Autodesk Inventor part; units mm, degrees
ref_plane "YZ Plane" through (0, 0, 0) normal (1, 0, 0) x (0, 1, 0)
ref_plane "XZ Plane" through (0, 0, 0) normal (0, 1, 0) x (-1, 0, 0)
ref_plane "XY Plane" through (0, 0, 0) normal (0, 0, 1) x (1, 0, 0)
sketch "Szkic1" plane through (0, 0, 0) normal (0, 1, 0) x (-1, 0, 0)
  line L0 (5.43, 11.8473) -> (13.43, 11.8473)
  line L1 (13.43, -12.1527) -> (-9.57, -12.1527)
  line L2 (-9.57, -12.1527) -> (-9.57, -27.1527)
  line L3 (-9.57, -27.1527) -> (-21.17, -27.1527)
  arc A0 (5.43, 11.8473) -> (3.5548, 10.5426) centre (5.43, 9.8473) ccw
  line L4 (3.5548, 10.5426) -> (-8.7625, -5.2144)
  arc A1 (-12.3382, -3.9827) -> (-8.7625, -5.2144) centre (-10.3382, -3.9827) ccw
  line L5 (-12.3382, -3.9827) -> (-12.3382, 0.0173)
  line L6 (-21.17, -27.1527) -> (-21.17, 0.0173)
  line L7 (-21.17, 0.0173) -> (-12.3382, 0.0173)
  line L8 (13.43, 11.8473) -> (13.43, 5.8473)
  line L9 (13.43, 5.8473) -> (9.43, 5.8473)
  line L10 (9.43, 5.8473) -> (9.43, 1.8473)
  line L11 (9.43, 1.8473) -> (13.43, 1.8473)
  line L12 (13.43, 1.8473) -> (13.43, -2.1527)
  line L13 (13.43, -2.1527) -> (9.43, -2.1527)
  line L14 (9.43, -2.1527) -> (9.43, -6.1527)
  line L15 (9.43, -6.1527) -> (13.43, -6.1527)
  line L16 (13.43, -6.1527) -> (13.43, -12.1527)
  point P0 (0, 0)
  dimension "d0" = 8
  dimension "d1" = 24
  dimension "d2" = 23
  dimension "d3" = 15
  dimension "d4" = 11.6
  dimension "d5" = 2
  dimension "d6" = 20
  dimension "d7" = 2
  dimension "d8" = 4
  dimension "d13" = 6
  dimension "d15" = 4
  dimension "d16" = 4
  dimension "d17" = 4
  dimension "d18" = 4
revolve "Obrót1" add sketch "Szkic1" angle 360 about axis through (21.17, 0, -27.1527) along (0, 0, 1)
sketch "Szkic2" plane through (21.17, 0, -27.1527) normal (0, 0, -1) x (-1, 0, 0)
  point P0 (21.17, 0)
sketch "Szkic3" plane through (21.17, 0, -27.1527) normal (0, 0, -1) x (-1, 0, 0)
  circle A0 centre (0, 0) radius 5
  point P0 (21.17, 0)
  dimension "d10" = 10
sketch "Szkic4" plane through (21.17, 0, -27.1527) normal (0, 0, -1) x (-1, 0, 0)
  point P0 (21.17, 0)
extrude "Wyciągnięcie proste1" cut sketch "Szkic3" against normal blind 39
properties part number "pierścień_uszczelniający" material "Tworzywo sztuczne PET"
The model under review builds one solid part; all positions refer to its coordinate system, in mm. A direction names the side the tool comes from. Round coordinates to 2 decimals unless told otherwise and drop trailing zeros. Order: outer loops, then holes, each group sorted by start corner. A loop starts at its lowest first (then second) coordinate and runs counter-clockwise, first axis right, second up. Notation, with made-up numbers: (-4.5, 21) -> (6.5, 21) arc R23 cw to (6.5, 49) -> close; hole circle Ø2 at (50, 45). An arc over 180 degrees is marked (long way). Write item = value, one per line. Start each with the question number.
Item 1: Consider section C-C on y = 28. Write out the cut boundary in (x, z).
Item 2: For line 1 along Z through (x, y) = (-6.5, 15); line 2 along Y through (x, z) = (21.5, -7.5); line 3 along Y through (x, z) = (21.17, -20), list the stretches that pass through material, from the lowest coordinate up.
Item 3: Consider section D-D on z = -14. Write out the cut boundary in (x, y), plus the area to 3 significant figures.
Item 4: Mouldability with a two-part tool opening along X and no side actions: class faces 1 (the face through (-11.832, 10.393, -9.195)), 2 (the face through (26.165, 0.22, -13.758)), 3 (the face through (19, 31, -2.153)) as released by +X, released by -X, zero draft, split by the parting line, or undercut.
Item 5: Clearance check with flat-ended pins moving along their axes: pin 1 Ø1.5 at (x, y) = (48, -19) entering from -Z; pin 2 Ø1 at (x, z) = (30.5, -6) entering from +Y; pin 3 Ø8 at (x, y) = (18, 18.5) entering from +Z. State where each tip first meets the part, or that it passes through.
Item 6: Consider section A-A on z = -1. Write out the cut boundary in (x, y).
Item 7: Consider section B-B on z = -8. Write out the cut boundary in (x, y).
Item 8: For faces 4 (the face through (45.453, -18.62, 3.819)), 5 (the face through (17, 4, 0.017)), 6 (the face through (-11.832, 10.393, 8.805)), 7 (the face through (11, 25, 11.847)), 8 (the face through (6, 0, -12.153)), list the 3-axis set-ups (+Z, -Z, +X, -X, +Y, -Y) from which the entire face can be reached by the end or side of a thin tool; tool diameter is ignored.
Conclusion:
q1.outline = (0.84, -12.15) -> (41.5, -12.15) -> (41.5, -6.15) -> (33.51, -6.15) -> (33.51, -2.15) -> (41.5, -2.15) -> (41.5, 1.85) -> (33.51, 1.85) -> (33.51, 5.85) -> (41.5, 5.85) -> (41.5, 11.85) -> (0.84, 11.85) -> (0.84, 5.85) -> (8.83, 5.85) -> (8.83, 1.85) -> (0.84, 1.85) -> (0.84, -2.15) -> (8.83, -2.15) -> (8.83, -6.15) -> (0.84, -6.15) -> close
q2.line_1 = -12.15 to -6.15, -2.15 to 1.85, 5.85 to 11.85
q2.line_2 = -34.6 to -4.99, 4.99 to 34.6
q2.line_3 = -11.6 to -5, 5 to 11.6
q3.outline = circle Ø23.2 at (21.17, 0); hole circle Ø10 at (21.17, 0)
q3.area = 344 mm2
q4.face_1 = split by the parting line
q4.face_2 = undercut
q4.face_3 = zero draft
q5.pin_1 = -12.15
q5.pin_2 = 33.45
q5.pin_3 = 8.04
q6.outline = circle Ø69.2 at (21.17, 0); circle Ø17.66 at (21.17, 0); hole circle Ø31.4 at (21.17, 0); hole circle Ø10 at (21.17, 0)
q7.outline = circle Ø69.2 at (21.17, 0); hole circle Ø10 at (21.17, 0)
q8.face_4 = none
q8.face_5 = +Z
q8.face_6 = +Z, -Z
q8.face_7 = +Z, +X, -X, +Y, -Y
q8.face_8 = -Z
